Check sheet for the modelled part. Datum: model origin and axes. Units: mm. Face numbers are marked on the shaded views. Round coordinates to 2 decimals unless told otherwise and drop trailing zeros. Loops run counter-clockwise (first coordinate to the right, second up) from the corner with the lowest first, then second, coordinate; pieces in that order, holes last. Notation, with made-up numbers: M -20.75,45 L -6.75,45 A19 ccw -6.75,69 Z; hole C -38,49.5 d11. An arc over 180 degrees is marked long. One line per question, with ' | ' between items. Start each with the question number.
(1) Section check D-D (x = 36). Record the boundary of the cut face in (y, z).
(2) Section check A-A (z = -78). Record the boundary of the cut face in (x, y).
(3) Section check B-B (z = 47.5). Record the boundary of the cut face in (x, y), and give its area (3 significant figures).
(4) Go/stop test with flat-tipped pins: P1, Ø3.5, axis at x = 42, y = -4, coming from the +Z side; P2, Ø6, axis at x = 52, z = 21, coming from the -Y side; P3, Ø5.5, axis at x = 75, y = 0, coming from the +Z side; P4, Ø5.5, axis at x = -75, z = -78, coming from the +Y side. Record where each tip stops, or that it passes through.
(5) Thickness scan on probe 1 along X at (y, z) = (4.5, 39); probe 2 along Y at (x, z) = (-75, 91.25); probe 3 along X at (y, z) = (-1.5, 59). Record the ranges inside material, lowest first. Write a range as [from, to].
(6) Draft check along X on the marked faces 1, 2 and 3. Enter one of: +X half, -X half, draft (parallel to the pull), parting line (faces both ways), or undercut.
(7) Section check C-C (x = -35.5). Record the boundary of the cut face in (y, z), and give its area (3 significant figures).
```python
from build123d import *

# Parameters (mm, degrees)
F0_W      = 200
F0_H      = 200
F1_DEPTH  = 10
F2_R      = 15
F3_DEPTH  = 20.001
F5_D      = 8.8
F7_DEPTH  = 20.001
F8_W      = 12
F8_H      = 130
F9_DEPTH  = 10
F10_R     = 10
F13_D     = 6.8
F13_DEPTH = 19.25
F13_TIP   = 2.0429261047


# Not quite as in the source:
# - two fillets or chamfers of one size are made in one step
# - a feature names something its author has since deleted; it is built from what else it names


with BuildPart() as f1:
    # F0 (on Front) → F1 (new body, symmetric)
    with BuildSketch(Plane.XZ):
        Rectangle(F0_W, F0_H)
    extrude(amount=F1_DEPTH, both=True)

    # F2 (on face) → F3 (cut, through all)
    with BuildSketch(Plane.XZ.offset(10)):
        Circle(F2_R)
    extrude(amount=-F3_DEPTH, mode=Mode.SUBTRACT)

    # F5 (through all)
    with Locations(Plane.XZ.offset(10)):
        with Locations((-75, -78), (75, -78)):
            Hole(F5_D / 2)

    # F6 (on face) → F7 (cut, through all)
    with BuildSketch(Plane.XZ.offset(10)):
        with BuildLine():
            Line((45, 100), (-45, 100))
            Line((-45, 100), (-45, -30))
            Line((-45, -30), (-40, -30))
            ThreePointArc((-40, -30), (0, -50), (40, -30))
            Line((40, -30), (45, -30))
            Line((45, -30), (45, 100))
        make_face()
    extrude(amount=-F7_DEPTH, mode=Mode.SUBTRACT)

    # F8 (on face) → F9 (cut)
    with BuildSketch(Plane.XZ.offset(10)):
        with Locations((-51, 35)):
            Rectangle(F8_W, F8_H)
        with Locations((51, 35)):
            Rectangle(F8_W, F8_H)
    extrude(amount=-F9_DEPTH, mode=Mode.SUBTRACT)

    # F10
    f10_edges = [f1.edges().sort_by_distance(p)[0] for p in [
        (-100, 0, 100),
        (-45, 5, 100),
        (45, 5, 100),
        (100, 0, 100),
        (100, 0, -100),
        (-100, 0, -100),
        (-57, -5, -30),
        (57, -5, -30),
    ]]
    fillet(f10_edges, radius=F10_R)

    # F13
    with Locations(Plane.XY.offset(100)):
        with Locations((-75, 0), (75, 0)):
            Hole(F13_D / 2, depth=F13_DEPTH)
            with Locations((0, 0, -(F13_DEPTH + F13_TIP / 2))):  # 118° drill point
                Cone(0, F13_D / 2, F13_TIP, mode=Mode.SUBTRACT)


solid = f1.part
```
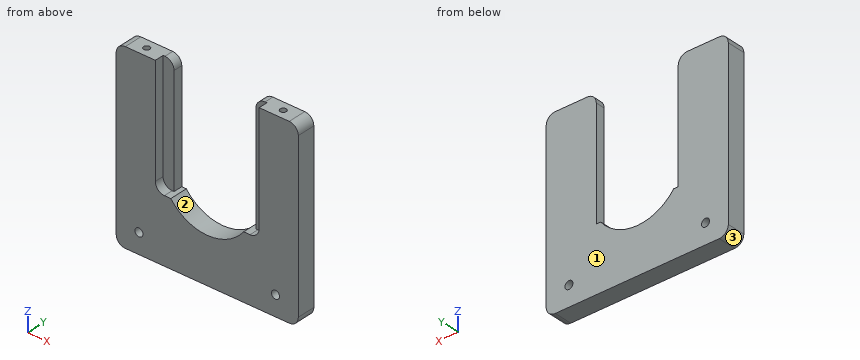
The answers:
1) outline: M -10,-100 L 10,-100 L 10,-34.7 L -10,-34.7 Z
2) outline: M -100,-10 L -79.4,-10 L -79.4,10 L -100,10 Z; M -70.6,-10 L 70.6,-10 L 70.6,10 L -70.6,10 Z; M 79.4,-10 L 100,-10 L 100,10 L 79.4,10 Z
3) outline: M -100,-10 L -57,-10 L -57,0 L -45,0 L -45,10 L -100,10 Z; M 45,0 L 57,0 L 57,-10 L 100,-10 L 100,10 L 45,10 Z | area: 1,960 mm²
4) P1: z = -30 | P2: y = 0 | P3: z = 80.36 | P4: through
5) probe 1: [-100, -45], [45, 100] | probe 2: [-10, -3.4], [3.4, 10] | probe 3: [-100, -57], [57, 100]
6) face 1: draft | face 2: undercut | face 3: -X half
7) outline: M -10,-100 L 10,-100 L 10,-35.21 L -10,-35.21 Z | area: 1,300 mm²
